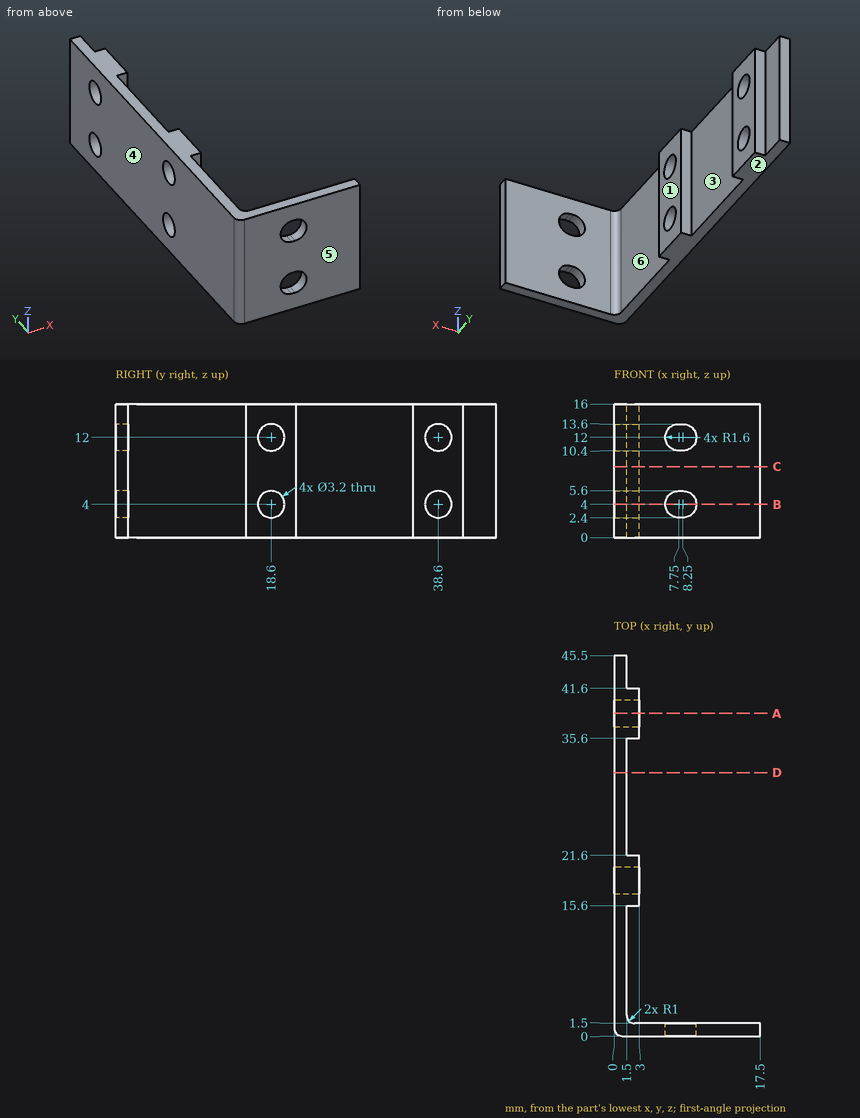
Could you check a few things on this drawing? It's one solid part, dimensions in mm from its lowest x, y, z. A direction names the side the tool comes from. Coordinates: 2 decimals unless noted, no trailing zeros. Write each loop counter-clockwise with the first axis right and the second up, starting at its lowest first coordinate (ties: lowest second). Pieces come first, ordered by that corner, then holes. Notation, with made-up numbers: (-24.5, -19) - (-15.5, -19) arc R21 ccw to (-15.5, 18) - close; hole circle Ø10 at (58, 78.25). An arc over 180 degrees is marked (long way). Put each result on its own line as item: value. Start each with the question number.
Q1. Which directions (+Z, -Z, +X, -X, +Y, -Y) give clear straight access to the entire face, cutting with the end or side of a thin tool? Please do the marked faces 1 and 2.
Q2. I'm going to push flat-ended pins straight in: P1, Ø5, axis at y = 18.6, z = 4, coming from the +X side; P2, Ø3, axis at x = 12, z = 6.5, coming from the +Y side; P3, Ø6.5, axis at y = 10, z = 10.5, coming from the +X side. Where does each tip first touch, or does it pass through?
Q3. I want a section at C-C on z = 8.5. Write out the boundary of the cut face in (x, y), plus the area to 3 significant figures.
Q4. I want a section at B-B on z = 4. Write out the boundary of the cut face in (x, y), plus the area to 3 significant figures.
Q5. Thinking about a two-plate mould opening in Y: for the marked faces 3, 4, 5 and 6, which applies, pulls with the +Y half, pulls with the -Y half, needs draft (parallel to the pull), parting line crosses it, or undercut?
Q6. I want a section at D-D on y = 31.5. Write out the boundary of the cut face in (x, z), plus the area to 3 significant figures.
Q7. I want a section at A-A on y = 38.6. Write out the boundary of the cut face in (x, z), plus the area to 3 significant figures.
Q8. Please list where these lines run through material, in increasing order: L1, parallel to Z at x = 0.85, y = 18.6; L2, parallel to Y at x = 2.5, z = 15.75; L3, parallel to Y at x = 14.25, z = 7.25.
Checks:
1. face 1: +Z, -Z, +X, +Y
1. face 2: -Z, +X, -X, +Y, -Y
2. P1: x = 3
2. P2: y = 1.5
2. P3: x = 1.5
3. outline: (0, 1) arc R1 ccw to (1, 0) - (17.5, 0) - (17.5, 1.5) - (2.5, 1.5) arc R1 cw to (1.5, 2.5) - (1.5, 15.6) - (3, 15.6) - (3, 21.6) - (1.5, 21.6) - (1.5, 35.6) - (3, 35.6) - (3, 41.6) - (1.5, 41.6) - (1.5, 45.5) - (0, 45.5) - close
3. area: 110 mm²
4. outline: (0, 1) arc R1 ccw to (1, 0) - (6.15, 0) - (6.15, 1.5) - (2.5, 1.5) arc R1 cw to (1.5, 2.5) - (1.5, 15.6) - (3, 15.6) - (3, 17) - (0, 17) - close; (0, 20.2) - (3, 20.2) - (3, 21.6) - (1.5, 21.6) - (1.5, 35.6) - (3, 35.6) - (3, 37) - (0, 37) - close; (0, 40.2) - (3, 40.2) - (3, 41.6) - (1.5, 41.6) - (1.5, 45.5) - (0, 45.5) - close; (9.85, 0) - (17.5, 0) - (17.5, 1.5) - (9.85, 1.5) - close
4. area: 85.5 mm²
5. face 3: undercut
5. face 4: needs draft
5. face 5: pulls with the -Y half
5. face 6: undercut
6. outline: (0, 0) - (1.5, 0) - (1.5, 16) - (0, 16) - close
6. area: 24.0 mm²
7. outline: (0, 0) - (3, 0) - (3, 2.4) - (0, 2.4) - close; (0, 5.6) - (3, 5.6) - (3, 10.4) - (0, 10.4) - close; (0, 13.6) - (3, 13.6) - (3, 16) - (0, 16) - close
7. area: 28.8 mm²
8. L1: 0 to 2.4, 5.6 to 10.4, 13.6 to 16
8. L2: 0 to 1.5, 15.6 to 21.6, 35.6 to 41.6
8. L3: 0 to 1.5
